```python
from build123d import *

# Parameters (mm, degrees)
F0_W      = 44.656470418
F0_H      = 33.8078811765
F1_DEPTH  = 16
F2_DEPTH  = 796
F3_DEPTH  = 196
F4_W      = 68.9578056335
F4_H      = 493.6993122101
F5_DEPTH  = 7
F6_DEPTH  = 9.7
F7_DEPTH  = 99.33
F8_DEPTH  = 99.33
F9_DEPTH  = 17.34
F10_DEPTH = 102.97
F11_W     = 35.2807044983
F11_H     = 492.0964837074
F12_DEPTH = 7
F13_DEPTH = 37.27
F14_DEPTH = 6.58
F15_DEPTH = 106.63
F16_DEPTH = 5.87
F17_DEPTH = 200
F18_DEPTH = 200
F19_DEPTH = 200
F20_DEPTH = 200
F21_DEPTH = 200
F22_DEPTH = 200
F23_DEPTH = 350
F24_DEPTH = 350
F25_DEPTH = 350
F26_R     = 3


with BuildPart() as f1:
    # F0 (on Front) → F1 (new body)
    with BuildSketch(Plane.XZ):
        with Locations((22.328235209, 16.9039405882)):
            Rectangle(F0_W, F0_H)
    extrude(amount=F1_DEPTH)

    # F2 (add): a face of the model
    f2_faces = [f1.faces().sort_by_distance(p)[0] for p in [
        (22.328235209, -8, 0),
    ]]
    extrude(f2_faces, amount=-F2_DEPTH)

    # F3 (add): a face of the model
    f3_faces = [f1.faces().sort_by_distance(p)[0] for p in [
        (0, -8, 398),
    ]]
    extrude(f3_faces, amount=-F3_DEPTH)

    # F4 (on face) → F5 (cut)
    with BuildSketch(Plane.XZ.offset(16)):
        with Locations((94.1769480705, 399.8196721077)):
            Rectangle(F4_W, F4_H)
    extrude(amount=-F5_DEPTH, mode=Mode.SUBTRACT)

    # F6 (cut): a face of the model
    f6_faces = [f1.faces().sort_by_distance(p)[0] for p in [
        (59.6980452538, -12.5, 399.8196721077),
    ]]
    extrude(f6_faces, amount=-F6_DEPTH, mode=Mode.SUBTRACT)

    # F7 (add): a face of the model
    f7_faces = [f1.faces().sort_by_distance(p)[0] for p in [
        (89.3269480705, -12.5, 646.6693282127),
    ]]
    extrude(f7_faces, amount=-F7_DEPTH)

    # F8 (cut): a face of the model
    f8_faces = [f1.faces().sort_by_distance(p)[0] for p in [
        (89.3269480705, -12.5, 646.6693282127),
    ]]
    extrude(f8_faces, amount=-F8_DEPTH, mode=Mode.SUBTRACT)

    # F9 (cut): a face of the model
    f9_faces = [f1.faces().sort_by_distance(p)[0] for p in [
        (128.6558508873, -12.5, 449.4846721077),
    ]]
    extrude(f9_faces, amount=-F9_DEPTH, mode=Mode.SUBTRACT)

    # F10 (cut): a face of the model
    f10_faces = [f1.faces().sort_by_distance(p)[0] for p in [
        (97.9969480705, -12.5, 152.9700160027),
    ]]
    extrude(f10_faces, amount=-F10_DEPTH, mode=Mode.SUBTRACT)

    # F11 (on face) → F12 (join)
    with BuildSketch(Plane.XZ.offset(9)):
        with Locations((91.7714834213, 432.6795041561)):
            Rectangle(F11_W, F11_H)
    extrude(amount=F12_DEPTH)

    # F13 (add): a face of the model
    f13_faces = [f1.faces().sort_by_distance(p)[0] for p in [
        (91.7714834213, -12.5, 678.7277460098),
    ]]
    extrude(f13_faces, amount=F13_DEPTH)

    # F14 (add): a face of the model
    f14_faces = [f1.faces().sort_by_distance(p)[0] for p in [
        (109.4118356705, -12.5, 451.3145041561),
    ]]
    extrude(f14_faces, amount=F14_DEPTH)

    # F15 (add): a face of the model
    f15_faces = [f1.faces().sort_by_distance(p)[0] for p in [
        (95.0614834213, -12.5, 186.6312623024),
    ]]
    extrude(f15_faces, amount=F15_DEPTH)

    # F16 (cut): a face of the model
    f16_faces = [f1.faces().sort_by_distance(p)[0] for p in [
        (74.1311311722, -12.5, 397.9995041561),
    ]]
    extrude(f16_faces, amount=-F16_DEPTH, mode=Mode.SUBTRACT)

    # F17 (add): a face of the model
    f17_faces = [f1.faces().sort_by_distance(p)[0] for p in [
        (196, -8, 398),
    ]]
    extrude(f17_faces, amount=F17_DEPTH)

    # F18 (cut): a face of the model
    f18_faces = [f1.faces().sort_by_distance(p)[0] for p in [
        (145.9958508873, -12.5, 397.9996721077),
    ]]
    extrude(f18_faces, amount=-F18_DEPTH, mode=Mode.SUBTRACT)

    # F19 (add): a face of the model
    f19_faces = [f1.faces().sort_by_distance(p)[0] for p in [
        (115.9918356705, -12.5, 397.9995041561),
    ]]
    extrude(f19_faces, amount=F19_DEPTH)

    # F20 (add): a face of the model
    f20_faces = [f1.faces().sort_by_distance(p)[0] for p in [
        (396, -8, 398),
    ]]
    extrude(f20_faces, amount=F20_DEPTH)

    # F21 (cut): a face of the model
    f21_faces = [f1.faces().sort_by_distance(p)[0] for p in [
        (345.9958508873, -12.5, 397.9996721077),
    ]]
    extrude(f21_faces, amount=-F21_DEPTH, mode=Mode.SUBTRACT)

    # F22 (add): a face of the model
    f22_faces = [f1.faces().sort_by_distance(p)[0] for p in [
        (315.9918356705, -12.5, 397.9995041561),
    ]]
    extrude(f22_faces, amount=F22_DEPTH)

    # F23 (cut): a face of the model
    f23_faces = [f1.faces().sort_by_distance(p)[0] for p in [
        (515.9918356705, -12.5, 397.9995041561),
    ]]
    extrude(f23_faces, amount=-F23_DEPTH, mode=Mode.SUBTRACT)

    # F24 (add): a face of the model
    f24_faces = [f1.faces().sort_by_distance(p)[0] for p in [
        (545.9958508873, -12.5, 397.9996721077),
    ]]
    extrude(f24_faces, amount=F24_DEPTH)

    # F25 (cut): a face of the model
    f25_faces = [f1.faces().sort_by_distance(p)[0] for p in [
        (596, -8, 398),
    ]]
    extrude(f25_faces, amount=-F25_DEPTH, mode=Mode.SUBTRACT)

    # F26
    f26_edges = [f1.edges().sort_by_distance(p)[0] for p in [
        (122.996483, -16, 715.997746),
        (165.991836, -16, 397.999504),
        (122.996483, -16, 80.001262),
        (80.001131, -16, 397.999504),
        (0, -16, 398),
        (123, -16, 796),
        (246, -16, 398),
        (123, -16, 0),
        (49.998045, -16, 397.999672),
        (122.996948, -16, 50.000016),
        (122.996948, -16, 745.999328),
        (195.995851, -16, 397.999672),
    ]]
    fillet(f26_edges, radius=F26_R)


solid = f1.part
```
For this review, take the finished solid that the model builds, in its own axes (mm). Round coordinates to 2 decimals unless told otherwise and drop trailing zeros. Write each loop counter-clockwise with the first axis right and the second up, starting at its lowest first coordinate (ties: lowest second). Pieces come first, ordered by that corner, then holes. Notation, with made-up numbers: (37, 66.5) - (89, 66.5) arc R26 ccw to (89, 87.5) - close; hole circle Ø10 at (-25.75, 60.5). An arc over 180 degrees is marked (long way). Answer as a JSON object with one key per item and string values.
1. To check wall thickness, follow line 1 along Z through (x, y) = (127, -9.5); line 2 along X through (y, z) = (-11.75, 166); line 3 along X through (y, z) = (-13.75, 581.5). State the ranges of each line that lie inside material, in increasing order.
Response values:
{"line 1": "z = 0 to 50, 80 to 716, 746 to 796", "line 2": "x = 0 to 50, 80 to 165.99, 196 to 246", "line 3": "x = 0.1 to 49.9, 80.1 to 165.9, 196.09 to 245.9"}
2. We need section A-A on z = 496.5. Give the boundary of the cut face in (x, y), then the cut area to 3 significant figures.
Response values:
{"outline": "(0, -13) arc R3 ccw to (3, -16) - (47, -16) arc R3 ccw to (50, -13) - (50, -9) - (80, -9) - (80, -13) arc R3 ccw to (83, -16) - (162.99, -16) arc R3 ccw to (165.99, -13) - (165.99, -9) - (196, -9) - (196, -13) arc R3 ccw to (199, -16) - (243, -16) arc R3 ccw to (246, -13) - (246, 0) - (0, 0) - close", "area": "3,500 mm2"}
3. Draft analysis for pull direction Z (two halves, no side actions). For faces 1 (the face through (121, 0, 404)), 2 (the face through (171, -9, 393)), 3 (the face through (121, -6, 0)), state which applies: +Z half, -Z half, draft (parallel to the pull), parting line (faces both ways), or undercut.
Response values:
{"face 1": "draft", "face 2": "undercut", "face 3": "-Z half"}
4. We need section B-B on x = 133.5. Give the boundary of the cut face in (y, z), then the cut area to 3 significant figures.
Response values:
{"outline": "(-16, 3) arc R3 ccw to (-13, 0) - (0, 0) - (0, 796) - (-13, 796) arc R3 ccw to (-16, 793) - (-16, 749) arc R3 ccw to (-13, 746) - (-9, 746) - (-9, 716) - (-13, 716) arc R3 ccw to (-16, 713) - (-16, 83) arc R3 ccw to (-13, 80) - (-9, 80) - (-9, 50) - (-13, 50) arc R3 ccw to (-16, 47) - close", "area": "12,300 mm2"}
